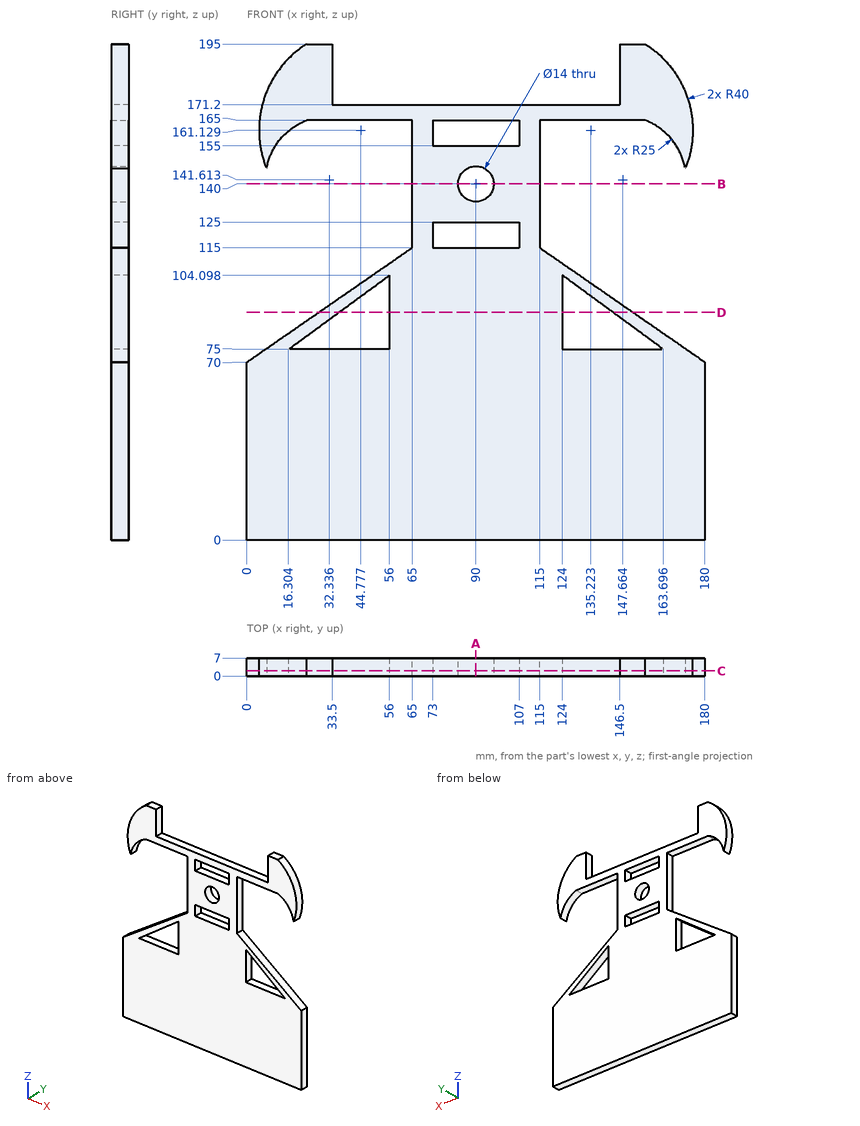
Design review of the part shown in the three views and the two pictorial views. Dimensions are in mm from the part's minimum x, y and z. Give positions to 0.01 mm unless a question says otherwise; leave off trailing zeros. Write each loop counter-clockwise with the first axis right and the second up, starting at its lowest first coordinate (ties: lowest second). Pieces come first, ordered by that corner, then holes.
Item 1: Take a section at C-C (y = 2). Give the number of separate pieces and of enclosed holes in the cut face, and give its area (3 significant figures).
Item 2: Take a section at D-D (z = 89.5). Give the boundary of the cut face in (x, y) (1 decimal), and give its area (3 significant figures).
Item 3: Insertion check: P1, Ø2, axis at y = 3.5, z = 147, coming from the -X side; P2, Ø3.5, axis at x = 96.5, y = 3.5, coming from the +Z side; P3, Ø12.5, axis at x = 90, z = 140, coming from the +Y side (3 decimals); P4, Ø3.5, axis at y = 3.5, z = 95, coming from the +X side (1 decimal). Each pin has a flat end and moves straight along its axis. Give the tip position at first contact, or say it passes through.
Item 4: Wall thickness on probe 1 along Z at (x, y) = (90, 5.75); probe 2 along Z at (x, y) = (97.5, 1); probe 3 along Z at (x, y) = (128.5, 3) (1 decimal): over which ranges is each line inside the solid? List them lowest first.
Item 5: Take a section at B-B (z = 140). Give the boundary of the cut face in (x, y).
Item 6: Take a section at A-A (x = 90). Give the boundary of the cut face in (y, z).
Established:
1. separate pieces: 1
1. enclosed holes: 5
1. area: 20,600 mm2
2. outline: (28.2, 0) - (36.1, 0) - (36.1, 7) - (28.2, 7) - close; (56, 0) - (124, 0) - (124, 7) - (56, 7) - close; (143.9, 0) - (151.8, 0) - (151.8, 7) - (143.9, 7) - close
2. area: 587 mm2
3. P1: stops at x = 6.99
3. P2: stops at z = 171.2
3. P3: passes through
3. P4: stops at x = 146.4
4. probe 1: z = 0 to 115, 125 to 133, 147 to 155, 165 to 171.2
4. probe 2: z = 0 to 115, 125 to 155, 165 to 171.2
4. probe 3: z = 0 to 75, 100.8 to 105.7, 165 to 171.2
5. outline: (65, 0) - (83, 0) - (83, 7) - (65, 7) - close; (97, 0) - (115, 0) - (115, 7) - (97, 7) - close
6. outline: (0, 0) - (7, 0) - (7, 115) - (0, 115) - close; (0, 125) - (7, 125) - (7, 133) - (0, 133) - close; (0, 147) - (7, 147) - (7, 155) - (0, 155) - close; (0, 165) - (7, 165) - (7, 171.2) - (0, 171.2) - close
